Autodesk Inventor part; units mm, degrees
ref_plane "YZ Plane" through (0, 0, 0) normal (1, 0, 0) x (0, 1, 0)
ref_plane "XZ Plane" through (0, 0, 0) normal (0, 1, 0) x (-1, 0, 0)
ref_plane "XY Plane" through (0, 0, 0) normal (0, 0, 1) x (1, 0, 0)
sketch "Sketch1" plane through (0, 0, 0) normal (0, 0, 1) x (1, 0, 0)
  line L0 (-40, 32.5) -> (40, 32.5)
  line L1 (40, 32.5) -> (40, -32.5)
  line L2 (40, -32.5) -> (-40, -32.5)
  line L3 (-40, -32.5) -> (-40, 32.5)
  line L4 (-40, 32.5) -> (40, -32.5) construction
  line L5 (40, 32.5) -> (-40, -32.5) construction
  line L6 (-8, 32.5) -> (-8, 24.5)
  line L7 (-8, 24.5) -> (-20, 24.5)
  line L8 (-20, 24.5) -> (-20, 28.5)
  line L9 (-20, 28.5) -> (-40, 28.5)
  line L10 (-40, -27) -> (-19, -27)
  line L11 (-19, -27) -> (-15.5, -23.5)
  line L12 (-15.5, -23.5) -> (-9.5, -23.5)
  line L13 (-9.5, -23.5) -> (-9.5, -32.5)
  line L14 (9.5, -32.5) -> (9.5, -23.5)
  line L15 (9.5, -23.5) -> (15.5, -23.5)
  line L16 (15.5, -23.5) -> (19, -27)
  line L17 (19, -27) -> (40, -27)
  point P0 (0, 0)
  dimension "d0" = 80
  dimension "d1" = 65
  dimension "d2" = 19
  dimension "d3" = 45
  dimension "d4" = 9
  dimension "d5" = 3.5
  dimension "d6" = 6
  dimension "d7" = 45
  dimension "d8" = 8
  dimension "d9" = 8
  dimension "d10" = 12
  dimension "d11" = 4
extrude "Extrusion1" add sketch "Sketch1" along normal blind 1.3 contours L0 L1 L17 L16 L15 L14 L2 L13 L12 L11 L10 L3 L9 L8 L7 L6
sketch "Sketch2" plane through (0, 0, 1.3) normal (0, 0, 1) x (1, 0, 0)
  line L0 (-35.7, -4.3) -> (35.7, -4.3) construction
  line L1 (-40, -27) -> (-19, -27)
  point P0 (0, 0)
  point P1 (0, -4.3)
  dimension "d14" = 71.4
  dimension "d15" = 22.7
hole "Hole1" at (-35.7, -4.3, 1.3) at (35.7, -4.3, 1.3) direction (0, 0, -1) diameter 2.5 end through all
sketch "Sketch4" plane through (-8, 32.5, 0) normal (0, 1, 0) x (1, 0, 0)
  line L0 (10.9, -2.9) -> (5.1, -2.9) construction
  line L1 (10.9, -1.3) -> (5.1, -1.3)
  line L2 (5.1, -4.5) -> (10.9, -4.5)
  arc A0 (10.9, -4.5) -> (10.9, -1.3) centre (10.9, -2.9) ccw
  arc A1 (5.1, -1.3) -> (5.1, -4.5) centre (5.1, -2.9) ccw
  line L3 (48, -1.3) -> (0, -1.3)
  line L4 (10.9, -2.9) -> (5.1, -2.9) construction
  line L5 (10.9, -1.7) -> (5.1, -1.7)
  line L6 (5.1, -4.1) -> (10.9, -4.1)
  arc A2 (10.9, -4.1) -> (10.9, -1.7) centre (10.9, -2.9) ccw
  arc A3 (5.1, -1.7) -> (5.1, -4.1) centre (5.1, -2.9) ccw
  point P0 (8, 0)
  point P1 (8, -2.9)
  point P2 (3.5, -2.9)
  point P3 (12.5, -2.9)
  point P4 (8, -2.9)
  dimension "d23" = 3.2
  dimension "d24" = 9
  dimension "d25" = 0.4
extrude "Extrusion2" add sketch "Sketch4" against normal blind 6.8
sketch "Sketch5" plane through (0, 0, 1.3) normal (0, 0, 1) x (1, 0, 0)
  circle A0 centre (-34.4, 23.1) radius 1.7
  circle A1 centre (34.4, 23.1) radius 1.7
  circle A2 centre (0, -22.3) radius 1.7
  line L0 (-34.4, 23.1) -> (34.4, 23.1) construction
  circle A3 centre (35.7, -4.3) radius 1.25
  point P0 (0, 0)
  point P1 (0, 23.1)
  dimension "d28" = 3.4
  dimension "d29" = 68.8
  dimension "d30" = 27.4
  dimension "d31" = 18
extrude "Extrusion3" add sketch "Sketch5" along normal blind 0.4 contours A0 | A1 | A2
sketch "Sketch6" plane through (0, -22.3, 1.7) normal (0, 0, 1) x (1, 0, 0)
  circle A0 centre (0, 0) radius 1.7
  circle A1 centre (-34.4, 45.4) radius 1.7
  circle A2 centre (34.4, 45.4) radius 1.7
  point P0 (0, 22.3)
extrude "Extrusion4" cut sketch "Sketch6" against normal through all
sketch "Sketch7" plane through (0, 0, 1.3) normal (0, 0, 1) x (1, 0, 0)
  line L0 (40, 32.5) -> (-8, 32.5)
  line L1 (40, 32.5) -> (40, 46.5)
  line L2 (40, 46.5) -> (-40, 46.5)
  line L3 (-40, 28.5) -> (-40, -27)
  line L4 (-40, 46.5) -> (-40, 28.5)
  line L5 (-40, 28.5) -> (-31, 28.5)
  line L6 (-20, 28.5) -> (-40, 28.5)
  line L7 (-31, 28.5) -> (-31, 37.5)
  line L8 (-31, 37.5) -> (31, 37.5)
  line L9 (31, 37.5) -> (31, 32.5)
  point P0 (0, 0)
  dimension "d36" = 9
  dimension "d37" = 9
  dimension "d38" = 9
  dimension "d39" = 5
extrude "Extrusion5" add sketch "Sketch7" against normal up to surface (1.3 mm away)
sketch "Sketch8" plane through (0, 0, 1.3) normal (0, 0, 1) x (1, 0, 0)
  line L0 (31, 32.5) -> (2.9, 32.5)
  line L1 (31, 32.5) -> (-31, 32.5)
  line L2 (-31, 32.5) -> (-31, -18.5)
  line L3 (-31, -18.5) -> (31, -18.5)
  line L4 (31, -18.5) -> (31, 32.5)
  line L5 (-31, 28.5) -> (-31, 37.5)
  line L6 (-15.5, -23.5) -> (-9.5, -23.5)
  line L7 (-40, -27) -> (-19, -27)
  line L8 (-15.5, -23.5) -> (-40, -23.5)
  line L9 (-40, -23.5) -> (-40, -27)
  line L10 (-40, -27) -> (-15.5, -27)
  line L11 (-15.5, -27) -> (-15.5, -23.5)
  line L12 (15.5, -23.5) -> (19, -27)
  line L13 (19, -27) -> (40, -27)
  line L14 (15.5, -23.5) -> (40, -23.5)
  line L15 (40, -23.5) -> (40, -27)
  line L16 (40, -27) -> (15.5, -27)
  line L17 (15.5, -27) -> (15.5, -23.5)
  line L18 (9.5, -32.5) -> (9.5, -23.5)
  line L19 (-9.5, -32.5) -> (9.5, -32.5)
  line L20 (9.5, -26.5) -> (-9.5, -26.5)
  line L21 (-9.5, -26.5) -> (-9.5, -32.5)
  line L22 (-9.5, -32.5) -> (9.5, -32.5)
  line L23 (9.5, -32.5) -> (9.5, -26.5)
  line L24 (-9.5, -23.5) -> (-9.5, -32.5)
  line L25 (-9.5, -23.5) -> (-4.5, -23.5)
  line L26 (-4.5, -23.5) -> (-4.5, -26.5)
  line L27 (-4.5, -26.5) -> (-9.5, -26.5)
  line L28 (-9.5, -26.5) -> (-9.5, -23.5)
  line L29 (9.5, -23.5) -> (15.5, -23.5)
  line L30 (9.5, -23.5) -> (4.5, -23.5)
  line L31 (4.5, -23.5) -> (4.5, -26.5)
  line L32 (4.5, -26.5) -> (9.5, -26.5)
  line L33 (9.5, -26.5) -> (9.5, -23.5)
  point P0 (0, 0)
  point P1 (-19, -27)
  point P2 (2.9, 32.5)
  dimension "d42" = 51
  dimension "d43" = 8
  dimension "d44" = 5
  dimension "d45" = 5
extrude "Extrusion6" cut sketch "Sketch8" against normal through all
sketch "Sketch9" plane through (-2.9, 32.5, 4.5) normal (0, 0, 1) x (1, 0, 0)
  line L0 (-5.3856, 3.3152) -> (10.2234, 3.3152)
  line L1 (10.2234, 3.3152) -> (10.2234, -11.8662)
  line L2 (10.2234, -11.8662) -> (-5.3856, -11.8662)
  line L3 (-5.3856, -11.8662) -> (-5.3856, 3.3152)
  point P0 (2.9, -32.5)
extrude "Extrusion7" cut sketch "Sketch9" against normal through all
fillet "Fillet1" radius 1 12 edges at (-31, 37.5, 0.65) (-40, 46.5, 0.65) (31, 37.5, 0.65) (40, 46.5, 0.65) (40, -23.5, 0.65) (31, -18.5, 0.65) (4.5, -23.5, 0.65) (4.5, -26.5, 0.65) (-4.5, -26.5, 0.65) (-4.5, -23.5, 0.65) (-31, -18.5, 0.65) (-40, -23.5, 0.65)
sketch "Sketch10" plane through (0, 0, 1.3) normal (0, 0, 1) x (1, 0, 0)
  line L0 (39, 46.5) -> (-39, 46.5)
  circle A0 centre (-35.7, -4.3) radius 1.25
  circle A1 centre (35.7, -4.3) radius 1.25
  line L1 (31, 36.5) -> (31, -17.5)
  arc A2 (30, -18.5) -> (31, -17.5) centre (30, -17.5) ccw
  line L2 (30, -18.5) -> (-30, -18.5)
  arc A3 (-31, -17.5) -> (-30, -18.5) centre (-30, -17.5) ccw
  line L3 (-31, -17.5) -> (-31, 36.5)
  arc A4 (-30, 37.5) -> (-31, 36.5) centre (-30, 36.5) ccw
  line L4 (-30, 37.5) -> (30, 37.5)
  arc A5 (31, 36.5) -> (30, 37.5) centre (30, 36.5) ccw
  circle A6 centre (0, -22.3) radius 1.7
  circle A7 centre (34.4, 23.1) radius 1.7
  circle A8 centre (-34.4, 23.1) radius 1.7
  arc A9 (-40, -22.5) -> (-39, -23.5) centre (-39, -22.5) ccw
  line L5 (-39, -23.5) -> (-5.5, -23.5)
  arc A10 (-4.5, -24.5) -> (-5.5, -23.5) centre (-5.5, -24.5) ccw
  line L6 (-4.5, -24.5) -> (-4.5, -25.5)
  arc A11 (-4.5, -25.5) -> (-3.5, -26.5) centre (-3.5, -25.5) ccw
  line L7 (-3.5, -26.5) -> (3.5, -26.5)
  arc A12 (3.5, -26.5) -> (4.5, -25.5) centre (3.5, -25.5) ccw
  line L8 (4.5, -25.5) -> (4.5, -24.5)
  arc A13 (5.5, -23.5) -> (4.5, -24.5) centre (5.5, -24.5) ccw
  line L9 (5.5, -23.5) -> (39, -23.5)
  arc A14 (39, -23.5) -> (40, -22.5) centre (39, -22.5) ccw
  line L10 (40, -22.5) -> (40, 45.5)
  arc A15 (40, 45.5) -> (39, 46.5) centre (39, 45.5) ccw
  line L11 (39, 46.5) -> (-39, 46.5)
  arc A16 (-39, 46.5) -> (-40, 45.5) centre (-39, 45.5) ccw
  line L12 (-40, 45.5) -> (-40, -22.5)
  point P0 (0, 0)
extrude "Extrusion8" add sketch "Sketch10" along normal blind 0.1
equation "\"d7\" = d3"
equation "\"d37\" = d36"
equation "\"d38\" = d36"
equation "\"d45\" = d44"
properties part number "PlacementTest"
Check sheet for the modelled part. Datum: model origin and axes. Units: mm. Give positions to 0.01 mm unless a question says otherwise; leave off trailing zeros. Write each loop counter-clockwise with the first axis right and the second up, starting at its lowest first coordinate (ties: lowest second). Pieces come first, ordered by that corner, then holes. Notation, with made-up numbers: (59, 80) - (80, 80) arc R20 ccw to (80, 118) - close; hole circle Ø10 at (40.25, -4). An arc over 180 degrees is marked (long way). Answer as a JSON object with one key per item and string values. Group by question number.
1) Thickness scan on probe 1 along X at (y, z) = (-4.3, 0.4); probe 2 along Y at (x, z) = (34.4, 0.95); probe 3 along Y at (x, z) = (-21, 0.65). Record the ranges inside material, lowest first. Write a range as from..to.
2) Sectioned sample at C-C (x = 29). Record the cut outline in (y, z).
3) Sectioned sample at D-D (y = 23.1). Record the cut outline in (x, z), then the cut area to 3 significant figures.
4) Sectioned sample at B-B (z = 1). Give the number of separate pieces and of enclosed holes in the cut face, then the cut area to 3 significant figures.
5) Release check for a two-part mould opening along X. For faces 1 (the face through (-1, 43, 1.4)), 2 (the face through (35.2, 21.6, 0.7)), 3 (the face through (-35.75, 22.07, 0.71)) record: pulls with the +X half, pulls with the -X half, needs draft (parallel to the pull), parting line crosses it, or undercut.
6) Sectioned sample at A-A (y = 14). Record the cut outline in (x, z).
7) Depth check by flat-ended pin: P1, Ø0.7, axis at x = 17.5, z = 1, coming from the -Y side. Enter the tip coordinate at first touch or a pass-through.
Geometry results:
{
 "1": {"probe 1": "x = -40..-36.95, -34.45..-31, 31..34.45, 36.95..40", "probe 2": "y = -23.5..21.4, 24.8..46.5", "probe 3": "y = -23.5..-18.5, 37.5..46.5"},
 "2": {"outline": "(-23.5, 0) - (-18.5, 0) - (-18.5, 1.4) - (-23.5, 1.4) - close; (37.5, 0) - (46.5, 0) - (46.5, 1.4) - (37.5, 1.4) - close"},
 "3": {"outline": "(-40, 0) - (-36.1, 0) - (-36.1, 1.4) - (-40, 1.4) - close; (-32.7, 0) - (-31, 0) - (-31, 1.4) - (-32.7, 1.4) - close; (31, 0) - (32.7, 0) - (32.7, 1.4) - (31, 1.4) - close; (36.1, 0) - (40, 0) - (40, 1.4) - (36.1, 1.4) - close", "area": "15.7 mm^2"},
 "4": {"separate pieces": "1", "enclosed holes": "6", "area": "2,120 mm^2"},
 "5": {"face 1": "needs draft", "face 2": "undercut", "face 3": "undercut"},
 "6": {"outline": "(-40, 0) - (-31, 0) - (-31, 1.4) - (-40, 1.4) - close; (31, 0) - (40, 0) - (40, 1.4) - (31, 1.4) - close"},
 "7": {"P1": "stops at y = -23.5"}
}
